Source: CAD feature listing. Evaluate the final solid. Frame: model axes, mm. Face numbers are marked on the shaded views. A direction names the side the tool comes from. Coordinates: 2 decimals unless noted, no trailing zeros. Order: outer loops, then holes, each group sorted by start corner. A loop starts at its lowest first (then second) coordinate and runs counter-clockwise, first axis right, second up. Notation, with made-up numbers: (43, 57.5) -> (94, 57.5) arc R22 cw to (94, 75.5) -> close; hole circle Ø10 at (37, 69). An arc over 180 degrees is marked (long way). Put each result on its own line as item: value.
from build123d import *

# Parameters (mm, degrees)
SKETCH1_R           = 4
BOSS_EXTRUDE1_DEPTH = 21
SKETCH2_R           = 3
CUT_EXTRUDE1_DEPTH  = 10
CUT_EXTRUDE3_START  = -10
SKETCH3_R           = 3
CUT_EXTRUDE3_DEPTH  = 10


with BuildPart() as part:
    # Sketch1 → Boss-Extrude1 (new body)
    with BuildSketch(Plane(origin=(0, 0, 0), x_dir=(1, 0, 0), z_dir=(0, 1, 0))):
        with Locations(Location((0, 0, 0), (0, 0, 90))):
            Circle(SKETCH1_R)
    extrude(amount=BOSS_EXTRUDE1_DEPTH)

    # Sketch2 → Cut-Extrude1 (cut)
    with BuildSketch(Plane.XZ):
        with Locations(Location((0, 0, 0), (0, 0, 270))):
            Circle(SKETCH2_R)
    extrude(amount=-CUT_EXTRUDE1_DEPTH, mode=Mode.SUBTRACT)

    # Sketch3 → Cut-Extrude3 (cut)
    with BuildSketch(Plane(origin=(0, 21, 0), x_dir=(1, 0, 0), z_dir=(0, 1, 0)).offset(CUT_EXTRUDE3_START)):
        with Locations(Location((0, 0, 0), (0, 0, 90))):
            Circle(SKETCH3_R)
    extrude(amount=CUT_EXTRUDE3_DEPTH, mode=Mode.SUBTRACT)

    # Cut-Extrude5: read off the stored shape, not the designer's step
    # Cut-Extrude5: loft between two sections, ruled curve by curve
    cut_extrude5_from = [
        Edge.make_three_point_arc((-2.653136305, 14.6, 0), (-2.653136305, 16, 1.4), (-2.653136305, 17.4, 0)),
        Edge.make_three_point_arc((-2.653136305, 17.4, 0), (-2.653136305, 16, -1.4), (-2.653136305, 14.6, 0)),
    ]
    cut_extrude5_to = [
        Edge.make_three_point_arc((-3.999916451, 14.6, 0), (-3.999916451, 16, 1.4), (-3.999916451, 17.4, 0)),
        Edge.make_three_point_arc((-3.999916451, 17.4, 0), (-3.999916451, 16, -1.4), (-3.999916451, 14.6, 0)),
    ]
    cut_extrude5 = Solid(Shell([*[Face.make_surface_from_curves(cut_extrude5_from[k], cut_extrude5_to[k]) for k in range(2)], Face(Wire(cut_extrude5_from)), Face(Wire(cut_extrude5_to))]))
    add(cut_extrude5, mode=Mode.SUBTRACT)

    # Cut-Extrude5 2: loft between two sections, ruled curve by curve
    cut_extrude5_2_from = [
        Edge.make_three_point_arc((-2.653136305, 3.6, 0), (-2.653136305, 5, 1.4), (-2.653136305, 6.4, 0)),
        Edge.make_three_point_arc((-2.653136305, 6.4, 0), (-2.653136305, 5, -1.4), (-2.653136305, 3.6, 0)),
    ]
    cut_extrude5_2_to = [
        Edge.make_three_point_arc((-3.999916451, 3.6, 0), (-3.999916451, 5, 1.4), (-3.999916451, 6.4, 0)),
        Edge.make_three_point_arc((-3.999916451, 6.4, 0), (-3.999916451, 5, -1.4), (-3.999916451, 3.6, 0)),
    ]
    cut_extrude5_2 = Solid(Shell([*[Face.make_surface_from_curves(cut_extrude5_2_from[k], cut_extrude5_2_to[k]) for k in range(2)], Face(Wire(cut_extrude5_2_from)), Face(Wire(cut_extrude5_2_to))]))
    add(cut_extrude5_2, mode=Mode.SUBTRACT)


solid = part.part
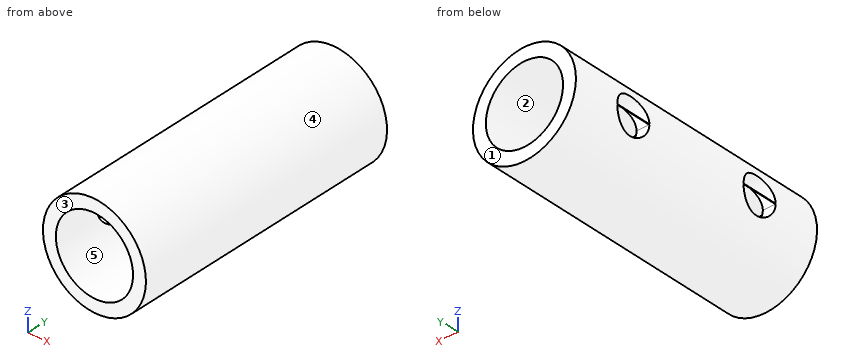
1. Cut plane A-A on x = 0. Output: boundary loops of the cut face in (y, z), plus the area to 3 significant figures.
Numbers:
outline: (0, -4) -> (21, -4) -> (21, -3) -> (11, -3) -> (11, 3) -> (21, 3) -> (21, 4) -> (0, 4) -> (0, 3) -> (10, 3) -> (10, -3) -> (0, -3) -> close
area: 48.0 mm2
2. Cut plane D-D on z = -0.5. Count the separate pieces of the cut face and the enclosed holes in it, plus the area to 3 significant figures.
Numbers:
separate pieces: 3
enclosed holes: 0
area: 43.1 mm2
3. First-contact query: pin 1 (1.5 mm diameter, centred on x = -3, y = 18, fed in from -Z). Flat tip, straight axial feed; report the tip coordinate or a pass-through.
Numbers:
pin 1: stops at z = -3.31
4. Ray query, line 1 along X through (y, z) = (6.5, 0); line 2 along Y through (x, z) = (-1.5, 1); line 3 along Z through (x, y) = (-2.5, 6.5). Return the intervals inside material, ascending.
Numbers:
line 1: x = -4 to -3, 3 to 4
line 2: y = 10 to 11
line 3: z = -3.12 to -1.66, 1.66 to 3.12
5. Pull-direction query (Z, two-part tool) for the marked faces 3, 4 and 5; classes: pulls with the +Z half, pulls with the -Z half, needs draft (parallel to the pull), parting line crosses it, or undercut.
Numbers:
face 3: needs draft
face 4: parting line crosses it
face 5: undercut
6. Cut plane B-B on y = 14. Output: boundary loops of the cut face in (x, z).
Numbers:
outline: circle Ø8 at (0, 0); hole circle Ø6 at (0, 0)
7. Set-up query: the marked faces 1 and 2. Return all of +Z, -Z, +X, -X, +Y, -Y with unobstructed straight access to the full face (end or side cutting, diameter ignored); none if empty.
Numbers:
face 1: +Z, -Z, +X, -X, +Y
face 2: +Y
8. Cut plane C-C on z = -2. Output: boundary loops of the cut face in (x, y).
Numbers:
outline: (-3.46, 0) -> (-2.24, 0) -> (-2.24, 10) -> (2.24, 10) -> (2.24, 0) -> (3.46, 0) -> (3.46, 21) -> (2.24, 21) -> (2.24, 11) -> (-2.24, 11) -> (-2.24, 21) -> (-3.46, 21) -> close
